from build123d import *

# Parameters (mm, degrees)
EXTRUDE_THIN1_DEPTH = 25
SKETCH2_R           = 2.5
CUT_EXTRUDE1_DEPTH  = 21
SKETCH3_R           = 2.5
CUT_EXTRUDE2_DEPTH  = 2.5


with BuildPart() as part:
    # Sketch1 → Extrude-Thin1 (new body)
    with BuildSketch(Plane.XY):
        Polygon((0, 20), (0, 0), (20, 0), (20, 1.5), (1.5, 1.5), (1.5, 20), align=None)
    extrude(amount=EXTRUDE_THIN1_DEPTH)

    # Sketch2 → Cut-Extrude1 (cut, through all)
    with BuildSketch(Plane(origin=(0, 0, 0), x_dir=(-1, 0, 0), z_dir=(0, -1, 0))):
        with Locations((-10, -5)):
            Circle(SKETCH2_R)
    extrude(amount=-CUT_EXTRUDE1_DEPTH, mode=Mode.SUBTRACT)

    # Sketch3 → Cut-Extrude2 (cut, through all)
    with BuildSketch(Plane(origin=(1.5, 0, 0), x_dir=(0, 0, -1), z_dir=(1, 0, 0))):
        with Locations((-20, 15)):
            Circle(SKETCH3_R)
    extrude(amount=-CUT_EXTRUDE2_DEPTH, mode=Mode.SUBTRACT)


solid = part.part
The model under review builds one solid part; all positions refer to its coordinate system, in mm. A direction names the side the tool comes from. Coordinates: 2 decimals unless noted, no trailing zeros. Order: outer loops, then holes, each group sorted by start corner. A loop starts at its lowest first (then second) coordinate and runs counter-clockwise, first axis right, second up. Notation, with made-up numbers: (-21.5, -32) -> (23.5, -32) arc R20 ccw to (23.5, -2) -> close; hole circle Ø9 at (33.5, -35). An arc over 180 degrees is marked (long way). Answer in a Markdown table with one row per item.
(1) Consider section B-B (z = 20). Write out the cut boundary in (x, y).
Answers:
| item | result |
|---|---|
| outline | (0, 0) -> (20, 0) -> (20, 1.5) -> (1.5, 1.5) -> (1.5, 12.5) -> (0, 12.5) -> close; (0, 17.5) -> (1.5, 17.5) -> (1.5, 20) -> (0, 20) -> close |
(2) Wall thickness on line 1 along X through (y, z) = (0.6, 5); line 2 along Y through (x, z) = (1, 20); line 3 along Z through (x, y) = (10, 1.1): over which ranges is each line inside the solid? List them lowest first.
Answers:
| item | result |
|---|---|
| line 1 | 0 to 7.5, 12.5 to 20 |
| line 2 | 0 to 12.5, 17.5 to 20 |
| line 3 | 0 to 2.5, 7.5 to 25 |
(3) Consider section C-C (x = 10). Write out the cut boundary in (y, z).
Answers:
| item | result |
|---|---|
| outline | (0, 0) -> (1.5, 0) -> (1.5, 2.5) -> (0, 2.5) -> close; (0, 7.5) -> (1.5, 7.5) -> (1.5, 25) -> (0, 25) -> close |
(4) Consider section A-A (y = 15). Write out the cut boundary in (x, z).
Answers:
| item | result |
|---|---|
| outline | (0, 0) -> (1.5, 0) -> (1.5, 17.5) -> (0, 17.5) -> close; (0, 22.5) -> (1.5, 22.5) -> (1.5, 25) -> (0, 25) -> close |
(5) The part is to be moulded in two halves that separate along Z. For faces 1 (the cylindrical face through (12.5, 0.7, 4.9)), 2 (the flat face through (1, 6, 0)), 3 (the flat face through (0, 10, 12)), say which applies: +Z half, -Z half, draft (parallel to the pull), parting line (faces both ways), or undercut.
Answers:
| item | result |
|---|---|
| face 1 | undercut |
| face 2 | -Z half |
| face 3 | draft |
(6) Consider section D-D (z = 15). Write out the cut boundary in (x, y), plus the area to 4 significant figures.
Answers:
| item | result |
|---|---|
| outline | (0, 0) -> (20, 0) -> (20, 1.5) -> (1.5, 1.5) -> (1.5, 20) -> (0, 20) -> close |
| area | 57.75 mm² |
(7) Machinability: for faces 4 (the cylindrical face through (0.8, 15.1, 22.5)), 5 (the flat face through (1.5, 11, 12)), which of the approach directions +Z, -Z, +X, -X, +Y, -Y give a long, thin tool a straight path to every point of the face, cutting with its end or side? Answer none if there is none.
Answers:
| item | result |
|---|---|
| face 4 | +X, -X |
| face 5 | +Z, -Z, +X, +Y |
(8) Insertion check: pin 1 (6 mm diameter, centred on x = 15.5, z = 7.5, fed in from +Y); pin 2 (10 mm diameter, centred on x = 8.5, z = 11, fed in from -Y); pin 3 (4 mm diameter, centred on y = 15, z = 20, fed in from -X). Each pin has a flat end and moves straight along its axis. Give the tip position at first contact, or say it passes through.
Answers:
| item | result |
|---|---|
| pin 1 | y = 1.5 |
| pin 2 | y = 0 |
| pin 3 | through |
